Drawing for the job (mm, zero at the part's lowest x, y, z). Round coordinates to 2 decimals unless told otherwise and drop trailing zeros. Order: outer loops, then holes, each group sorted by start corner. A loop starts at its lowest first (then second) coordinate and runs counter-clockwise, first axis right, second up. Notation, with made-up numbers: (57.25, -10) -> (71.25, -10) arc R6 cw to (71.25, -4) -> close; hole circle Ø2 at (71, -28). An arc over 180 degrees is marked (long way). Answer as CSV lines item,"result". Start each with the question number.
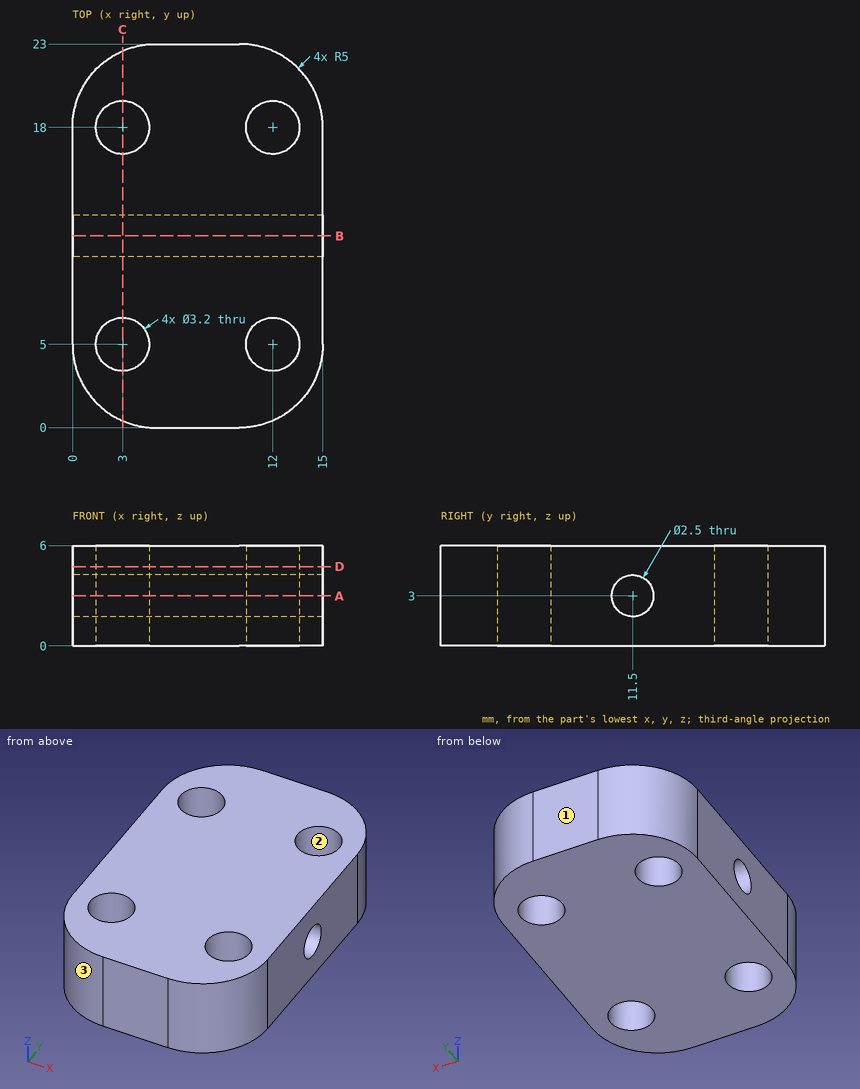
Q1. Slice it at C-C, the plane x = 3. Write the cut outline in (y, z), plus the area to 3 significant figures.
Q2. Probe L1, parallel to Z at x = 6, y = 11.5; L2, parallel to Y at x = 3, z = 1.35; L3, parallel to Y at x = 12, z = 3.7. List the from-to ranges inside material, lowest first.
Q3. Slice it at B-B, the plane y = 11.5. Write the cut outline in (x, z), plus the area to 3 significant figures.
Q4. Two-plate mould, pull along X, no slides. Class the marked faces 1, 2 and 3: +X half, -X half, draft (parallel to the pull), parting line (faces both ways), or undercut.
Q5. Slice it at A-A, the plane z = 3. Write the cut outline in (x, y), plus the area to 3 significant figures.
Q6. Flat gauge pin, fed straight in: pin 1 Ø3 at (x, y) = (3, 5) entering from +Z. Where does the tip first touch, or does it go through?
Q7. Slice it at D-D, the plane z = 4.75. Write the cut outline in (x, y).
Solutions:
1,outline,"(0.42, 0) -> (3.4, 0) -> (3.4, 6) -> (0.42, 6) -> close; (6.6, 0) -> (16.4, 0) -> (16.4, 6) -> (6.6, 6) -> close; (19.6, 0) -> (22.58, 0) -> (22.58, 6) -> (19.6, 6) -> close; hole circle Ø2.5 at (11.5, 3)"
1,area,"89.7 mm2"
2,L1,"z = 0 to 1.75, 4.25 to 6"
2,L2,"y = 0.42 to 3.4, 6.6 to 16.4, 19.6 to 22.58"
2,L3,"y = 0.42 to 3.4, 6.6 to 10.46, 12.54 to 16.4, 19.6 to 22.58"
3,outline,"(0, 0) -> (15, 0) -> (15, 1.75) -> (0, 1.75) -> close; (0, 4.25) -> (15, 4.25) -> (15, 6) -> (0, 6) -> close"
3,area,"52.5 mm2"
4,face 1,"draft"
4,face 2,"undercut"
4,face 3,"-X half"
5,outline,"(0, 5) arc R5 ccw to (5, 0) -> (10, 0) arc R5 ccw to (15, 5) -> (15, 10.25) -> (0, 10.25) -> close; (0, 12.75) -> (15, 12.75) -> (15, 18) arc R5 ccw to (10, 23) -> (5, 23) arc R5 ccw to (0, 18) -> close; hole circle Ø3.2 at (3, 5); hole circle Ø3.2 at (3, 18); hole circle Ø3.2 at (12, 5); hole circle Ø3.2 at (12, 18)"
5,area,"254 mm2"
6,pin 1,"passes through"
7,outline,"(0, 5) arc R5 ccw to (5, 0) -> (10, 0) arc R5 ccw to (15, 5) -> (15, 18) arc R5 ccw to (10, 23) -> (5, 23) arc R5 ccw to (0, 18) -> close; hole circle Ø3.2 at (3, 5); hole circle Ø3.2 at (3, 18); hole circle Ø3.2 at (12, 5); hole circle Ø3.2 at (12, 18)"
